Solid Edge part; units mm, degrees
sketch "Sketch1" plane through (0, 0, 0) normal (0, 0, 1) x (1, 0, 0)
  circle A0 centre (-6.75, 75.7107) radius 1.5
  circle A1 centre (6.75, 75.7107) radius 1.5
  line L0 (-9.75, 57.4107) -> (-21.25, 57.4107)
  line L1 (-21.25, 57.4107) -> (-21.25, 35.4107)
  line L2 (-21.25, 35.4107) -> (-9.75, 35.4107)
  line L3 (-9.75, 57.4107) -> (-9.75, 35.4107)
  circle A2 centre (17.7673, 40.9107) radius 1.5
  line L4 (50, -50) -> (50, 0)
  arc A3 (50, 0) -> (70.5719, -4.4281) centre (50, -50) cw
  arc A4 (70.5719, -4.4281) -> (49.5699, 50.4264) centre (0, 0) ccw
  arc A5 (-49.5699, 50.4264) -> (49.5699, 50.4264) centre (0, 24.5274) cw
  arc A6 (-70.5719, -4.4281) -> (-49.5699, 50.4264) centre (0, 0) cw
  arc A7 (-50, 0) -> (-70.5719, -4.4281) centre (-50, -50) ccw
  line L5 (-50, 0) -> (-50, -50)
  arc A8 (-50, -50) -> (50, -50) centre (0, 0) ccw
  dimension "D1" = 21.25
  dimension "D2" = 21.25
extrude "Protrusion1" add sketch "Sketch1" along normal blind 3
sketch "Sketch2" plane through (0, 4.8723, 0) normal (0, 0, -1) x (0, 1, 0)
  circle A0 centre (55.2883, -15.5) radius 1
  circle A1 centre (27.7883, -15.5) radius 1
  line L0 (25.0383, -6.5) -> (58.0383, -6.5)
  line L1 (58.0383, -6.5) -> (58.0383, -24.5)
  line L2 (58.0383, -24.5) -> (25.0383, -24.5)
  line L3 (25.0383, -24.5) -> (25.0383, -6.5)
extrude "ExtrudedProtrusion_2" add sketch "Sketch2" along normal blind 5
sketch "Sketch3" plane through (-15.5, 46.4107, 0) normal (0, 0, 1) x (1, 0, 0)
  line L0 (-5.75, 11) -> (5.75, 11)
  line L1 (5.75, 11) -> (5.75, -11)
  line L2 (5.75, -11) -> (-5.75, -11)
  line L3 (-5.75, -11) -> (-5.75, 10.8886)
extrude "Cutout1" cut sketch "Sketch3" against normal blind 126.1563 material side at (-15.5, 57.3607, 0)
sketch "Sketch4" plane through (0, 4.8723, 3) normal (0, 0, 1) x (0, 1, 0)
  circle A0 centre (-65.2277, 0) radius 1.5
  circle A1 centre (6.4136, 60.2859) radius 1.5
  circle A2 centre (6.4136, -60.2859) radius 1.5
extrude "ExtrudedProtrusion_3" add sketch "Sketch4" along normal blind 3
sketch "Sketch5" plane through (0, 4.8723, 0) normal (0, 0, -1) x (0, -1, 0)
  circle A0 centre (-6.4136, 60.2859) radius 1.5
  circle A1 centre (-6.4136, -60.2859) radius 1.5
extrude "ExtrudedCutout_3" cut sketch "Sketch5" against normal blind 1394.131
sketch "Sketch6" plane through (0, 4.8723, 0) normal (0, 0, -1) x (0, -1, 0)
  circle A0 centre (65.2277, 0) radius 1.5
extrude "ExtrudedCutout_4" cut sketch "Sketch6" against normal blind 239.0862
sketch "Sketch7" plane through (0, 4.8723, 3) normal (0, 0, 1) x (0, -1, 0)
  circle A0 centre (-55.2883, -15.5) radius 1
  circle A1 centre (-27.7883, -15.5) radius 1
extrude "ExtrudedCutout_5" cut sketch "Sketch7" against normal blind 54.4855
Input: part model. Units: mm. Frame: model coordinates. A direction names the side the tool comes from. Round coordinates to 2 decimals unless told otherwise and drop trailing zeros. Loops run counter-clockwise (first coordinate to the right, second up) from the corner with the lowest first, then second, coordinate; pieces in that order, holes last. Notation, with made-up numbers: (-3.5, 80.5) -> (3.5, 80.5) arc R29 cw to (3.5, 103.5) -> close; hole circle Ø3 at (24.5, -22.75). An arc over 180 degrees is marked (long way). Answer as a JSON object with one key per item and string values. Group by question number.
1) Section query B-B on z = 1.75. State how many separate pieces and enclosed holes the cut face has, plus the area to 3 significant figures.
2) Section query D-D on x = 43.5. Output: boundary loops of the cut face in (y, z), plus the area to 3 significant figures.
3) Pin query (flat end, axial travel): pin 1 (4 mm diameter, centred on x = -16, z = 0.5, fed in from +Y); pin 2 (2.5 mm diameter, centred on y = 42.5, z = -2.5, fed in from +X); pin 3 (2.5 mm diameter, centred on x = -20, z = -1.5, fed in from +Y). Return the tip coordinate at first contact, or that it passes through.
4) Ray query, L1, parallel to Y at x = -15.5, z = -2.5; L2, parallel to X at y = 37.5, z = -1.5; L3, parallel to X at y = 61.5, z = -0.25. Return the intervals inside material, ascending.
5) Section query C-C on y = -36. Output: boundary loops of the cut face in (x, z), plus the area to 3 significant figures.
6) Reachability of faces 4 (the cylindrical face through (-60.67, -1.15, 1.48)), 5 (the flat face through (-9.75, 47, -1)), 6 (the flat face through (-16, 29.911, -2)), 7 (the flat face through (-15, 62.911, -2)) from +Z, -Z, +X, -X, +Y, -Y: full face, straight path, thin tool, end or side. Return the list, or none.
7) Section query A-A on x = -11.5. Output: boundary loops of the cut face in (y, z).
8) Draft query along X for faces 1 (the cylindrical face through (60.38, -1.09, 1.48)), 2 (the flat face through (-24.5, 47, -2)), 3 (the cylindrical face through (-0.85, 80.45, 1.48)). Return one class per face: +X half, -X half, draft (parallel to the pull), parting line (faces both ways), or undercut.
Reply:
{
 "1": {"separate pieces": "1", "enclosed holes": "9", "area": "14,800 mm2"},
 "2": {"outline": "(-55.75, 0) -> (59.68, 0) -> (59.68, 3) -> (-55.75, 3) -> close", "area": "346 mm2"},
 "3": {"pin 1": "stops at y = 78.67", "pin 2": "stops at x = -6.5", "pin 3": "stops at y = 62.91"},
 "4": {"L1": "y = 29.91 to 31.66, 33.66 to 35.41, 57.41 to 59.16, 61.16 to 62.91", "L2": "x = -24.5 to -21.25, -9.75 to -6.5", "L3": "x = -24.5 to -6.5"},
 "5": {"outline": "(-50, 0) -> (50, 0) -> (50, 3) -> (-50, 3) -> close", "area": "300 mm2"},
 "6": {"face 4": "+Z, -Z, -Y", "face 5": "+Z, -Z", "face 6": "-Z, +X, -X, -Y", "face 7": "-Z, +X, -X, +Y"},
 "7": {"outline": "(-69.77, 0) -> (29.91, 0) -> (29.91, -5) -> (35.41, -5) -> (35.41, 3) -> (-69.77, 3) -> close; (57.41, -5) -> (62.91, -5) -> (62.91, 0) -> (79.26, 0) -> (79.26, 3) -> (57.41, 3) -> close"},
 "8": {"face 1": "undercut", "face 2": "-X half", "face 3": "parting line"}
}
